Autodesk Fusion 360 part; units mm, degrees
sketch "Esquisse1" plane through (0, 0, 0) normal (0, 0, 1) x (1, 0, 0)
  line L0 (74.4967, -39.3812) -> (-42.7033, -39.3812)
  line L1 (-42.7033, 30.8188) -> (74.4967, 30.8188)
  line L2 (76.4967, 28.8188) -> (76.4967, -37.3812)
  line L3 (-44.7033, -37.3812) -> (-44.7033, 28.8188)
  arc A0 (76.4967, 28.8188) -> (74.4967, 30.8188) centre (74.4967, 28.8188) ccw
  arc A1 (-42.7033, 30.8188) -> (-44.7033, 28.8188) centre (-42.7033, 28.8188) ccw
  arc A2 (-44.7033, -37.3812) -> (-42.7033, -39.3812) centre (-42.7033, -37.3812) ccw
  arc A3 (74.4967, -39.3812) -> (76.4967, -37.3812) centre (74.4967, -37.3812) ccw
  point P0 (-37.2797, 0.2421)
  point P1 (-65.57, -27.6552)
  dimension "d25" = 121.2
  dimension "d26" = 70.2
  dimension "d31" = 2
  dimension "d32" = 2
  dimension "d33" = 2
  dimension "d34" = 2
extrude "Extrusion1" add sketch "Esquisse1" along normal blind 47
sketch "Esquisse2" plane through (0, 0, 47) normal (0, 0, 1) x (-1, 0, 0)
  arc A0 (44.7033, 37.3812) -> (42.7033, 39.3812) centre (42.7033, 37.3812) ccw
  line L0 (42.7033, 39.3812) -> (-74.4967, 39.3812)
  arc A1 (-74.4967, 39.3812) -> (-76.4967, 37.3812) centre (-74.4967, 37.3812) ccw
  line L1 (-76.4967, 37.3812) -> (-76.4967, -28.8188)
  arc A2 (-76.4967, -28.8188) -> (-74.4967, -30.8188) centre (-74.4967, -28.8188) ccw
  line L2 (-74.4967, -30.8188) -> (42.7033, -30.8188)
  arc A3 (42.7033, -30.8188) -> (44.7033, -28.8188) centre (42.7033, -28.8188) ccw
  line L3 (44.7033, -28.8188) -> (44.7033, 37.3812)
  line L4 (39.7033, -25.8188) -> (39.7033, 34.3812)
  line L5 (39.7033, 34.3812) -> (-71.4967, 34.3812)
  line L6 (-71.4967, 34.3812) -> (-71.4967, -25.8188)
  line L7 (-71.4967, -25.8188) -> (39.7033, -25.8188)
  line L8 (42.2033, -28.3188) -> (42.2033, 36.8812)
  line L9 (42.2033, 36.8812) -> (-73.9967, 36.8812)
  line L10 (-73.9967, 36.8812) -> (-73.9967, -28.3188)
  line L11 (-73.9967, -28.3188) -> (42.2033, -28.3188)
  dimension "d37" = -2.5
  dimension "d49" = -5
extrude "Extrusion2" cut sketch "Esquisse2" against normal blind 1 contours L4 L5 L6 L7 | L8 L9 L10 L11
extrude "Extrusion4" cut sketch "Esquisse2" against normal blind 45 contours L4 L5 L6 L7
sketch "Esquisse3" plane through (76.4967, 0, 0) normal (1, 0, 0) x (0, 1, 0)
  line L0 (-37.3812, 0) -> (28.8188, 0)
  line L1 (28.8188, 0) -> (28.8188, 47)
  line L2 (28.8188, 47) -> (-37.3812, 47)
  line L3 (-37.3812, 47) -> (-37.3812, 0)
  line L4 (6.8188, 19) -> (24.8188, 19)
  line L5 (24.8188, 19) -> (24.8188, 4)
  line L6 (24.8188, 4) -> (6.8188, 4)
  line L7 (6.8188, 4) -> (6.8188, 19)
  dimension "d40" = 18
  dimension "d42" = 19
  dimension "d44" = 4
  dimension "d47" = 15
extrude "Extrusion3" cut sketch "Esquisse3" against normal blind 50 contours L4 L5 L6 L7
sketch "Esquisse4" plane through (0, -39.3812, 0) normal (0, -1, 0) x (1, 0, 0)
  line L0 (-42.7033, 0) -> (74.4967, 0)
  line L1 (74.4967, 0) -> (74.4967, 47)
  line L2 (74.4967, 47) -> (-42.7033, 47)
  line L3 (-42.7033, 47) -> (-42.7033, 0)
  line L4 (-0.5033, 12) -> (11.4967, 12)
  line L5 (11.4967, 12) -> (11.4967, 3)
  line L6 (11.4967, 3) -> (-0.5033, 3)
  line L7 (-0.5033, 3) -> (-0.5033, 12)
  dimension "d52" = 12
  dimension "d53" = 9
  dimension "d54" = 75
  dimension "d55" = 3
extrude "Extrusion5" cut sketch "Esquisse4" against normal blind 25 contours L4 L5 L6 L7
The listing builds one solid part. Answer for the finished solid, in the listing's coordinates (mm). A direction names the side the tool comes from. Give positions to 0.01 mm unless a question says otherwise; leave off trailing zeros. Order: outer loops, then holes, each group sorted by start corner. A loop starts at its lowest first (then second) coordinate and runs counter-clockwise, first axis right, second up.
1) Find section B-B on z = 38. Write down the section's boundary in (x, y), then the cut area to 3 significant figures.
Reported:
outline: (-44.7, -37.38) arc R2 ccw to (-42.7, -39.38) - (74.5, -39.38) arc R2 ccw to (76.5, -37.38) - (76.5, 28.82) arc R2 ccw to (74.5, 30.82) - (-42.7, 30.82) arc R2 ccw to (-44.7, 28.82) - close; hole (-39.7, -34.38) - (71.5, -34.38) - (71.5, 25.82) - (-39.7, 25.82) - close
area: 1,810 mm2
2) For faces 1 (the face through (15, -4, 0)), 2 (the face through (15, -34.381, 24)), 3 (the face through (74, 16, 4)), 4 (the face through (76.497, -4, 23)), 5 (the face through (11.497, -37, 8)), determine the directions among +Z, -Z, +X, -X, +Y, -Y from which every point of the face is accessible in a straight line to the end or side of a thin tool.
Reported:
face 1: -Z, +X, -X, +Y, -Y
face 2: +Z
face 3: +X
face 4: +Z, -Z, +X, +Y, -Y
face 5: -Y
3) Determine the mould class of faces 6 (the face through (17, -5, 2)), 7 (the face through (-0.503, -37, 7)), 8 (the face through (15, 30.819, 23)), 9 (the face through (17, -39.381, 23)) for opening direction Y: pulls with the +Y half, pulls with the -Y half, needs draft (parallel to the pull), parting line crosses it, or undercut.
Reported:
face 6: undercut
face 7: needs draft
face 8: pulls with the +Y half
face 9: pulls with the -Y half
4) Find section D-D on y = -28. Write down the section's boundary in (x, z).
Reported:
outline: (-44.7, 0) - (76.5, 0) - (76.5, 47) - (74, 47) - (74, 46) - (71.5, 46) - (71.5, 2) - (-39.7, 2) - (-39.7, 46) - (-42.2, 46) - (-42.2, 47) - (-44.7, 47) - close
5) Find section A-A on z = 5.5. Write down the section's boundary in (x, y), then the cut area to 3 significant figures.
Reported:
outline: (-44.7, -37.38) arc R2 ccw to (-42.7, -39.38) - (-0.5, -39.38) - (-0.5, -34.38) - (-39.7, -34.38) - (-39.7, 25.82) - (71.5, 25.82) - (71.5, 24.82) - (76.5, 24.82) - (76.5, 28.82) arc R2 ccw to (74.5, 30.82) - (-42.7, 30.82) arc R2 ccw to (-44.7, 28.82) - close; (11.5, -39.38) - (74.5, -39.38) arc R2 ccw to (76.5, -37.38) - (76.5, 6.82) - (71.5, 6.82) - (71.5, -34.38) - (11.5, -34.38) - close
area: 1,660 mm2
6) Find section C-C on x = 25.5. Write down the section's boundary in (y, z), then the cut area to 3 significant figures.
Reported:
outline: (-39.38, 0) - (30.82, 0) - (30.82, 47) - (28.32, 47) - (28.32, 46) - (25.82, 46) - (25.82, 2) - (-34.38, 2) - (-34.38, 46) - (-36.88, 46) - (-36.88, 47) - (-39.38, 47) - close
area: 585 mm2
7) Consider line 1 along X through (y, z) = (-7, 17); line 2 along Y through (x, z) = (-29, 27); line 3 along Z through (x, y) = (69.5, 0). Determine where each line is inside the solid, lowest interval first.
Reported:
line 1: x = -44.7 to -39.7, 71.5 to 76.5
line 2: y = -39.38 to -34.38, 25.82 to 30.82
line 3: z = 0 to 2
